from build123d import *

# Parameters (mm, degrees)
F0_W      = 120
F0_H      = 55
F0_R      = 2
F1_DEPTH  = 3
F2_W      = 1.125
F2_H      = 55
F3_DEPTH  = 6
F5_DEPTH  = 55
F6_W      = 0.4
F6_H      = 6
F7_DEPTH  = 56.2
F9_DEPTH  = 3
F10_SIZE  = 8
F11_W     = 9.086206
F11_H     = 67.30528
F11_W_2   = 12.61974
F11_H_2   = 69.156178
F12_DEPTH = 12.5


with BuildPart() as f1:
    # F0 (on Top) → F1 (new body)
    with BuildSketch(Plane.XY):
        Rectangle(F0_W, F0_H)
        with Locations((-30, -15)):
            Circle(F0_R, mode=Mode.SUBTRACT)
        with Locations((30, -15)):
            Circle(F0_R, mode=Mode.SUBTRACT)
        with Locations((-30, 15)):
            Circle(F0_R, mode=Mode.SUBTRACT)
        with Locations((30, 15)):
            Circle(F0_R, mode=Mode.SUBTRACT)
    extrude(amount=F1_DEPTH)

    # F2 (on face) → F3 (join)
    with BuildSketch(Plane.XY.offset(3)):
        with Locations((59.4375, 0)):
            Rectangle(F2_W, F2_H)
        with Locations((-59.4375, 0)):
            Rectangle(F2_W, F2_H)
    extrude(amount=F3_DEPTH)

    # F4 (on face) → F5 (join)
    with BuildSketch(Plane.XZ.offset(27.5)):
        Polygon((-52.744724, 0), (-58.875, 3), (-58.875, 9), (-55.875, 9), (-55.875, 11.75), (-61.875, 11.75), (-61.875, 0), align=None)
        Polygon((61.875, 11.75), (55.875, 11.75), (55.875, 9), (58.875, 9), (58.875, 3), (52.744724, 0), (61.875, 0), align=None)
    extrude(amount=-F5_DEPTH)

    # F6 (on face) → F7 (cut)
    with BuildSketch(Plane.XZ.offset(27.5)):
        with Locations((-59.075, 6)):
            Rectangle(F6_W, F6_H)
        with Locations((59.075, 6)):
            Rectangle(F6_W, F6_H)
    extrude(amount=-F7_DEPTH, mode=Mode.SUBTRACT)

    # F8 (on face) → F9 (join)
    with BuildSketch(Plane.XZ.offset(27.5)):
        Polygon((0, 3), (-55.875, 11.75), (-61.875, 11.75), (-61.875, 0), (61.875, 0), (61.875, 11.75), (55.875, 11.75), align=None)
    extrude(amount=-F9_DEPTH)

    # F10
    f10_edges = [f1.edges().sort_by_distance(p)[0] for p in [
        (58.875, 27.5, 11.75),
        (-58.875, 27.5, 11.75),
    ]]
    chamfer(f10_edges, length=F10_SIZE)

    # F11 (on face) → F12 (cut, symmetric)
    with BuildSketch(Plane.XY.offset(3)):
        with Locations((-65.543103, -0.961821)):
            Rectangle(F11_W, F11_H)
        with Locations((67.30987, -1.382478)):
            Rectangle(F11_W_2, F11_H_2)
    extrude(amount=F12_DEPTH, both=True, mode=Mode.SUBTRACT)


solid = f1.part
Work out the finished part from the listing and answer in its coordinate system (mm). A direction names the side the tool comes from. Round coordinates to 2 decimals unless told otherwise and drop trailing zeros. Write each loop counter-clockwise with the first axis right and the second up, starting at its lowest first coordinate (ties: lowest second). Pieces come first, ordered by that corner, then holes. Notation, with made-up numbers: M -29,58 L -5,58 A34 ccw -5,97 Z; hole C -20,10 d5. An arc over 180 degrees is marked long. Use a Markdown table: item, result.
1) The part is cut by section D-D on z = 7.5. Give the vertices of the cut face in (x, y) (3 decimals).
Taken from the geometry:
| item | result |
|---|---|
| outline | M -61,-27.5 L -28.736,-27.5 L -28.736,-24.5 L -59.275,-24.5 L -59.275,23.75 L -61,23.75 Z; M 28.736,-27.5 L 61,-27.5 L 61,23.75 L 59.275,23.75 L 59.275,-24.5 L 28.736,-24.5 Z |
2) Determine the mould class of faces 1 (the face through (58, -1, 9)), 2 (the face through (-1, -27.5, 2)), 3 (the face through (-1, 0, 0)) for opening direction Z: pulls with the +Z half, pulls with the -Z half, needs draft (parallel to the pull), parting line crosses it, or undercut.
Taken from the geometry:
| item | result |
|---|---|
| face 1 | undercut |
| face 2 | needs draft |
| face 3 | pulls with the -Z half |
3) Which of the six approach directions +Z, -Z, +X, -X, +Y, -Y give full straight-line access (tool end or side, diameter ignored) to faces 4 (the face through (-27.546, -26.021, 7.314)), 5 (the face through (61, 0, 6)), 6 (the face through (-58, -4, 11.75)), 7 (the face through (-59.275, 1, 6)), 8 (the face through (55.875, -1, 10))?
Taken from the geometry:
| item | result |
|---|---|
| face 4 | +Z, +Y, -Y |
| face 5 | +Z, -Z, +X, +Y, -Y |
| face 6 | +Z, +X, -X, +Y, -Y |
| face 7 | +Y |
| face 8 | +Z, +Y |
4) The part is cut by section A-A on y = -15. Give the vertices of the cut face in (x, z) (3 decimals), plus the area to 3 significant figures.
Taken from the geometry:
| item | result |
|---|---|
| outline | M -61,0 L -32,0 L -32,3 L -59.275,3 L -59.275,9 L -55.875,9 L -55.875,11.75 L -61,11.75 Z; M -28,0 L 28,0 L 28,3 L -28,3 Z; M 32,0 L 61,0 L 61,11.75 L 55.875,11.75 L 55.875,9 L 59.275,9 L 59.275,3 L 32,3 Z |
| area | 391 mm2 |
5) Consider line 1 (Y direction, x = -30, z = 1.45); line 2 (X direction, y = 19.5, z = 5.5) (3 decimals); line 3 (Z direction, x = 56.5, y = -18). Determine where each line is inside the solid, lowest interval first. Write a range as [from, to].
Taken from the geometry:
| item | result |
|---|---|
| line 1 | y = [-27.5, -17], [-13, 13], [17, 27.5] |
| line 2 | x = [-61, -59.275], [59.275, 61] |
| line 3 | z = [0, 3], [9, 11.75] |
6) Flat-ended cylindrical pins translate along their axes: pin 1 (3 mm diameter, centred on x = 30, y = -15, fed in from -Z); pin 2 (6 mm diameter, centred on x = -28, z = 7.5, fed in from +Y); pin 3 (5 mm diameter, centred on x = 30, y = 15, fed in from +Z). Find the tip coordinate at first contact, or state that the pin passes through.
Taken from the geometry:
| item | result |
|---|---|
| pin 1 | passes through |
| pin 2 | stops at y = -24.5 |
| pin 3 | stops at z = 3 |
7) The part is cut by section B-B on y = 24. Give the vertices of the cut face in (x, z) (3 decimals), plus the area to 3 significant figures.
Taken from the geometry:
| item | result |
|---|---|
| outline | M -61,0 L 61,0 L 61,7.25 L 59.275,7.25 L 59.275,3 L -59.275,3 L -59.275,7.25 L -61,7.25 Z |
| area | 381 mm2 |
8) The part is cut by section C-C on x = 30. Give the vertices of the cut face in (y, z), plus the area to 3 significant figures.
Taken from the geometry:
| item | result |
|---|---|
| outline | M -27.5,0 L -17,0 L -17,3 L -24.5,3 L -24.5,7.7 L -27.5,7.7 Z; M -13,0 L 13,0 L 13,3 L -13,3 Z; M 17,0 L 27.5,0 L 27.5,3 L 17,3 Z |
| area | 155 mm2 |
